For this review, take the finished solid that the model builds, in its own axes (mm). A direction names the side the tool comes from. Coordinates: 2 decimals unless noted, no trailing zeros. Loops run counter-clockwise (first coordinate to the right, second up) from the corner with the lowest first, then second, coordinate; pieces in that order, holes last.
1. Take a section at B-B, the plane z = -6.25. State the section outline as (x, y) points.
2. Take a section at A-A, the plane x = 6. State the section outline as (y, z) points.
3. To check wall thickness, follow probe 1 along Y at (x, z) = (4, -5.75); probe 2 along X at (y, z) = (6.75, -6.25); probe 3 along X at (y, z) = (20.75, -7). State the ranges of each line that lie inside material, in increasing order.
4. Mouldability with a two-part tool opening along Y and no side actions: class faces 1 (the face through (-1.1, 6, -6)), 2 (the face through (6, 2, -6)), 3 (the face through (6.4, 12, -6)), 4 (the face through (6, 23.4, -6)) as pulls with the +Y half, pulls with the -Y half, needs draft (parallel to the pull), parting line crosses it, or undercut.
5. Take a section at D-D, the plane z = -7.75. State the section outline as (x, y) points.
6. Take a section at C-C, the plane y = 21. State the section outline as (x, z) points, then the cut area to 3 significant figures.
7. Machinability: for faces 5 (the face through (7, 13, -11.7)), 6 (the face through (3, 9.5, -8)), which of the approach directions +Z, -Z, +X, -X, +Y, -Y give a long, thin tool a straight path to every point of the face, cutting with its end or side? Answer none if there is none.
8. Clearance check with a flat-ended pin moving along its axis: P1, Ø3, axis at y = 11.5, z = -7, coming from the -X side. State where the tip first meets the part, or that it passes through.
```python
from build123d import *

# Parameters (mm, degrees)
BOSS_EXTRUDE4_DEPTH = 25.4
SKETCH3_R           = 2
CUT_EXTRUDE1_DEPTH  = 25.4
SKETCH5_W           = 54.299093249
SKETCH5_H           = 94.215662961
CUT_EXTRUDE2_DEPTH  = 4.5
SKETCH7_W           = 18.693193774
SKETCH7_H           = 5.5
CUT_EXTRUDE3_DEPTH  = 14.5
SKETCH9_W           = 36.111652001
SKETCH9_H           = 33.164105193
CUT_EXTRUDE4_DEPTH  = 1
SKETCH10_W          = 62.791660767
SKETCH10_H          = 37.243179947
CUT_EXTRUDE6_DEPTH  = 1
FILLET2_R           = 3
SKETCH11_W          = 10.7
SKETCH11_H          = 5.5
BOSS_EXTRUDE5_DEPTH = 2
SKETCH12_W          = 13.41826103
SKETCH12_H          = 56.552103836
CUT_EXTRUDE7_DEPTH  = 10
SKETCH14_W          = 10.7
SKETCH14_H          = 5.5
BOSS_EXTRUDE7_DEPTH = 2
SKETCH15_W          = 10.7
SKETCH15_H          = 9.5
BOSS_EXTRUDE8_DEPTH = 6
SKETCH16_W          = 10.7
SKETCH16_H          = 10.4
BOSS_EXTRUDE9_DEPTH = 6
FILLET3_R           = 3
SKETCH18_W          = 10.7
SKETCH18_H          = 5.5
CUT_EXTRUDE8_DEPTH  = 1
SKETCH21_W          = 35.797160714
SKETCH21_H          = 35.29022369
CUT_EXTRUDE9_DEPTH  = 3
SKETCH22_W          = 25.937316652
SKETCH22_H          = 36.458252548
CUT_EXTRUDE10_DEPTH = 2
SKETCH23_W          = 31.218703754
SKETCH23_H          = 37.872657663
CUT_EXTRUDE11_DEPTH = 2
SKETCH24_R          = 2
CUT_EXTRUDE12_DEPTH = 24


with BuildPart() as part:
    # Sketch1 → Boss-Extrude4 (new body)
    with BuildSketch(Plane(origin=(0, 0, 0), x_dir=(1, 0, 0), z_dir=(0, 1, 0))):
        with BuildLine():
            Line((0.717280831, 0), (0, 0))
            Line((0, 0), (0, 9.078373892))
            ThreePointArc((0, 9.078373892), (-0.063231401, 9.104565196), (-0.089422705, 9.167796597))
            Line((-0.089422705, 9.167796597), (-0.089422705, 9.317189397))
            ThreePointArc((-0.089422705, 9.317189397), (-0.063231401, 9.380420798), (0, 9.406612102))
            Line((0, 9.406612102), (0, 12.7))
            Line((0, 12.7), (0.98359831, 12.7))
            ThreePointArc((0.98359831, 12.7), (-3.239897706, 11.634417694), (-5.100024486, 7.695723417))
            Line((-5.100024486, 7.695723417), (-5.100024486, 5.049332428))
            ThreePointArc((-5.100024486, 5.049332428), (-3.343059972, 1.197813276), (0.717280831, 0))
        make_face()
        with BuildLine():
            Line((0, 9.078373892), (0, 0))
            Line((0, 0), (0.717280831, 0))
            ThreePointArc((0.717280831, 0), (3.851519152, 1.706272455), (5.100024486, 5.049332428))
            Line((5.100024486, 5.049332428), (5.100024486, 7.695723417))
            ThreePointArc((5.100024486, 7.695723417), (3.938694277, 10.935621123), (0.98359831, 12.7))
            Line((0.98359831, 12.7), (0, 12.7))
            Line((0, 12.7), (0, 9.406612102))
            ThreePointArc((0, 9.406612102), (0.063231401, 9.380420798), (0.089422705, 9.317189397))
            Line((0.089422705, 9.317189397), (0.089422705, 9.167796597))
            ThreePointArc((0.089422705, 9.167796597), (0.063231401, 9.104565196), (0, 9.078373892))
        make_face()
        with BuildLine():
            ThreePointArc((5.100024486, 5.049332428), (3.851519152, 1.706272455), (0.717280831, 0))
            Line((0.717280831, 0), (20.32, 0))
            Line((20.32, 0), (20.32, 12.7))
            Line((20.32, 12.7), (0.98359831, 12.7))
            ThreePointArc((0.98359831, 12.7), (3.938694277, 10.935621123), (5.100024486, 7.695723417))
            Line((5.100024486, 7.695723417), (5.100024486, 5.049332428))
        make_face()
    extrude(amount=BOSS_EXTRUDE4_DEPTH)

    # Sketch3 → Cut-Extrude1 (cut)
    with BuildSketch(Plane(origin=(0, 25.4, 0), x_dir=(1, 0, 0), z_dir=(0, 1, 0))):
        with Locations(Location((0, 6.163356084, 0), (0, 0, 270))):
            Circle(SKETCH3_R)
    extrude(amount=-CUT_EXTRUDE1_DEPTH, mode=Mode.SUBTRACT)

    # Sketch5 → Cut-Extrude2 (cut)
    with BuildSketch(Plane(origin=(20.32, 0, 0), x_dir=(0, 0, -1), z_dir=(1, 0, 0))):
        with Locations((11.125522758, -8.280714776)):
            Rectangle(SKETCH5_W, SKETCH5_H)
    extrude(amount=-CUT_EXTRUDE2_DEPTH, mode=Mode.SUBTRACT)

    # Sketch7 → Cut-Extrude3 (cut)
    with BuildSketch(Plane.ZY.offset(5.100024486)):
        with Locations((-6.318501351, 12.25)):
            Rectangle(SKETCH7_W, SKETCH7_H)
    extrude(amount=-CUT_EXTRUDE3_DEPTH, mode=Mode.SUBTRACT)

    # Sketch9 → Cut-Extrude4 (cut)
    with BuildSketch(Plane(origin=(0, 0, -12.7), x_dir=(-1, 0, 0), z_dir=(0, 0, -1))):
        with Locations((-4.511590843, 12.177462725)):
            Rectangle(SKETCH9_W, SKETCH9_H)
    extrude(amount=-CUT_EXTRUDE4_DEPTH, mode=Mode.SUBTRACT)


with BuildPart() as body_2:
    # of the pieces the cut leaves, the one that is kept (cut_extrude4_keep)
    add(part.part.solids().sort_by_distance((-0.089422705, 0, -9.167796597))[0])

    # Sketch10 → Cut-Extrude6 (cut)
    with BuildSketch(Plane.XY):
        with Locations((3.132657463, 10.976513171)):
            Rectangle(SKETCH10_W, SKETCH10_H)
    extrude(amount=-CUT_EXTRUDE6_DEPTH, mode=Mode.SUBTRACT)


with BuildPart() as body_2_2:
    # of the pieces the cut leaves, the one that is kept (cut_extrude6_keep)
    add(body_2.part.solids().sort_by_distance((-0.089422705, 0, -9.167796597))[0])

    # Fillet2
    fillet2_edges = [body_2_2.edges().sort_by_distance(p)[0] for p in [
        (-3.100509095, 20.2, -1),
        (-3.100509095, 4.75, -1),
        (-3.158483624, 4.75, -11.7),
        (-3.158483624, 20.2, -11.7),
    ]]
    fillet(fillet2_edges, radius=FILLET2_R)

    # Sketch11 → Boss-Extrude5 (add)
    with BuildSketch(Plane.ZY.offset(-9.399975514)):
        with Locations((-6.35, 12.25)):
            Rectangle(SKETCH11_W, SKETCH11_H)
    extrude(amount=BOSS_EXTRUDE5_DEPTH)

    # Sketch12 → Cut-Extrude7 (cut)
    with BuildSketch(Plane.ZY.offset(5.100024486)):
        with Locations((-6.709130515, 16.674143704)):
            Rectangle(SKETCH12_W, SKETCH12_H)
    extrude(amount=-CUT_EXTRUDE7_DEPTH, mode=Mode.SUBTRACT)

    # Sketch14 → Boss-Extrude7 (add)
    with BuildSketch(Plane.ZY.offset(-7.399975514)):
        with Locations((-6.35, 12.25)):
            Rectangle(SKETCH14_W, SKETCH14_H)
    extrude(amount=BOSS_EXTRUDE7_DEPTH)

    # Sketch15 → Boss-Extrude8 (add)
    with BuildSketch(Plane.ZY.offset(-4.899975514)):
        with Locations((-6.35, 4.75)):
            Rectangle(SKETCH15_W, SKETCH15_H)
    extrude(amount=BOSS_EXTRUDE8_DEPTH)

    # Sketch16 → Boss-Extrude9 (add)
    with BuildSketch(Plane.ZY.offset(-4.899975514)):
        with Locations((-6.35, 20.2)):
            Rectangle(SKETCH16_W, SKETCH16_H)
    extrude(amount=BOSS_EXTRUDE9_DEPTH)

    # Fillet3
    fillet3_edges = [body_2_2.edges().sort_by_distance(p)[0] for p in [
        (-1.100024486, 4.75, -11.7),
        (-1.100024486, 4.75, -1),
        (-1.100024486, 20.2, -11.7),
        (-1.100024486, 20.2, -1),
    ]]
    fillet(fillet3_edges, radius=FILLET3_R)

    # Sketch18 → Cut-Extrude8 (cut)
    with BuildSketch(Plane.ZY.offset(-5.399975514)):
        with Locations((-6.35, 12.25)):
            Rectangle(SKETCH18_W, SKETCH18_H)
    extrude(amount=-CUT_EXTRUDE8_DEPTH, mode=Mode.SUBTRACT)

    # Sketch21 → Cut-Extrude9 (cut)
    with BuildSketch(Plane(origin=(15.82, 0, 0), x_dir=(0, 0, -1), z_dir=(1, 0, 0))):
        with Locations((4.247356295, 13.050264646)):
            Rectangle(SKETCH21_W, SKETCH21_H)
    extrude(amount=-CUT_EXTRUDE9_DEPTH, mode=Mode.SUBTRACT)

    # Sketch22 → Cut-Extrude10 (cut)
    with BuildSketch(Plane(origin=(0, 25.4, 0), x_dir=(1, 0, 0), z_dir=(0, 1, 0))):
        with Locations((4.63538262, 4.299284276)):
            Rectangle(SKETCH22_W, SKETCH22_H)
    extrude(amount=-CUT_EXTRUDE10_DEPTH, mode=Mode.SUBTRACT)

    # Sketch23 → Cut-Extrude11 (cut)
    with BuildSketch(Plane.XZ):
        with Locations((9.360738883, -6.802201309)):
            Rectangle(SKETCH23_W, SKETCH23_H)
    extrude(amount=-CUT_EXTRUDE11_DEPTH, mode=Mode.SUBTRACT)

    # Sketch24 → Cut-Extrude12 (cut)
    with BuildSketch(Plane.XZ.offset(-2)):
        with Locations(Location((1.599975514, -6.25, 0), (0, 0, 270))):
            Circle(SKETCH24_R)
    extrude(amount=-CUT_EXTRUDE12_DEPTH, mode=Mode.SUBTRACT)


solid = body_2_2.part
```
Results list:
1. outline: (-1.1, 2) - (-0.4, 2) - (-0.4, 9.5) - (-1.1, 9.5) - close; (-1.1, 15) - (-0.4, 15) - (-0.4, 23.4) - (-1.1, 23.4) - close; (3.6, 2) - (12.82, 2) - (12.82, 23.4) - (3.6, 23.4) - (3.6, 15) - (6.4, 15) - (6.4, 9.5) - (3.6, 9.5) - close
2. outline: (2, -11.7) - (9.5, -11.7) - (9.5, -1) - (2, -1) - close; (15, -11.7) - (23.4, -11.7) - (23.4, -1) - (15, -1) - close
3. probe 1: y = 2 to 9.5, 15 to 23.4
3. probe 2: x = -1.1 to -0.4, 3.6 to 12.82
3. probe 3: x = -1.1 to -0.25, 3.45 to 12.82
4. face 1: needs draft
4. face 2: pulls with the -Y half
4. face 3: undercut
4. face 4: pulls with the +Y half
5. outline: (-1.1, 2) - (0.28, 2) - (0.28, 9.5) - (-1.1, 9.5) - close; (-1.1, 15) - (0.28, 15) - (0.28, 23.4) - (-1.1, 23.4) - close; (2.92, 2) - (12.82, 2) - (12.82, 23.4) - (2.92, 23.4) - (2.92, 15) - (6.4, 15) - (6.4, 9.5) - (2.92, 9.5) - close
6. outline: (-1.1, -8.7) arc R3 ccw to (1.9, -11.7) - (12.82, -11.7) - (12.82, -1) - (1.9, -1) arc R3 ccw to (-1.1, -4) - close; hole circle Ø4 at (1.6, -6.25)
6. area: 133 mm2
7. face 5: -Z, +X, -X, +Y, -Y
7. face 6: +Z, -Z, -X
8. P1: stops at x = 6.4
